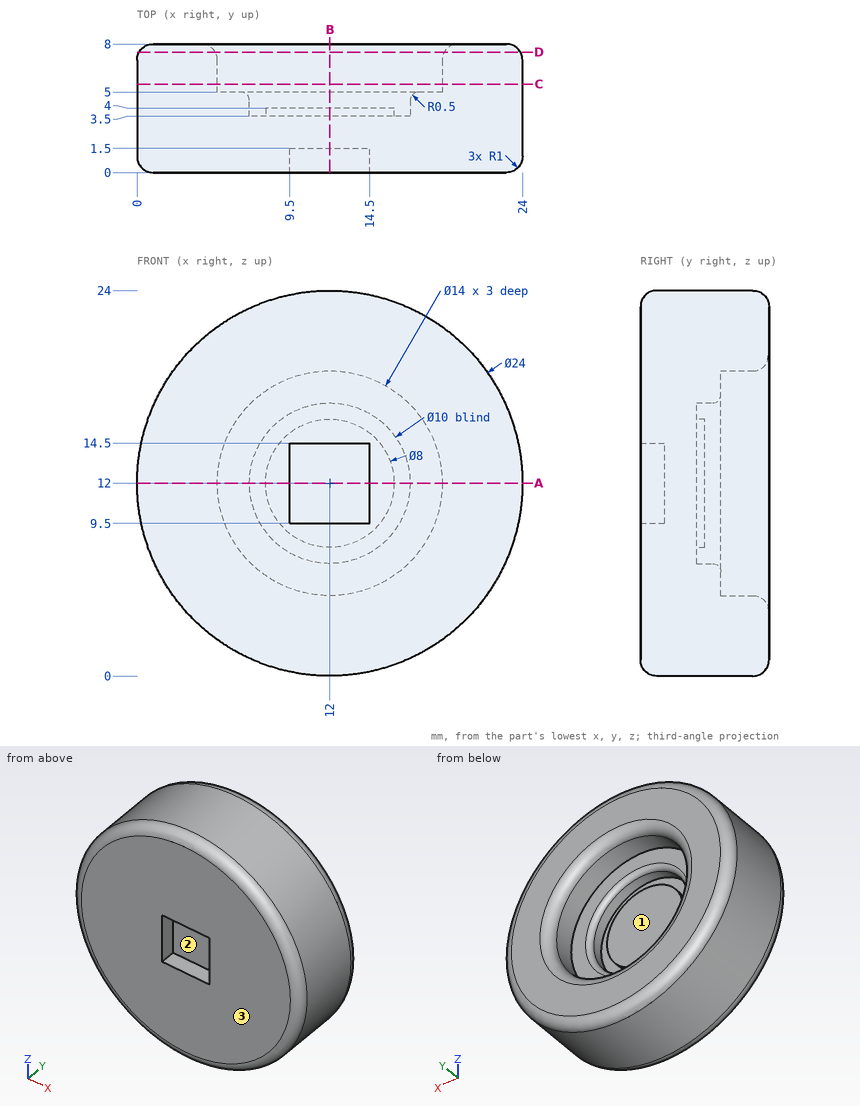
Input: dimensioned drawing with shaded views. Units: mm. Origin: part minimum x, y, z. A direction names the side the tool comes from. Coordinates: 2 decimals unless noted, no trailing zeros. Order: outer loops, then holes, each group sorted by start corner. A loop starts at its lowest first (then second) coordinate and runs counter-clockwise, first axis right, second up.
(1) Section query A-A (z = 12). Return the cut outline in (x, y), plus the area to 3 significant figures.
(2) Section query C-C (y = 5.5). Return the cut outline in (x, z), plus the area to 3 significant figures.
(3) Material intervals for probe 1 along X at (y, z) = (3.8, 12); probe 2 along Z at (x, y) = (12, 5.5), sorted ascending.
(4) Section query D-D (y = 7.5). Return the cut outline in (x, z).
(5) First-contact query: pin 1 (4 mm diameter, centred on x = 12, z = 10.5, fed in from +Y); pin 2 (2 mm diameter, centred on x = 13.5, z = 7, fed in from +Y); pin 3 (1.5 mm diameter, centred on y = 3.5, z = 17.5, fed in from +X). Flat tips, straight axial feed; report the tip coordinate or a pass-through.
(6) Access query for the marked faces 1, 2 and 3. Directions: +Z, -Z, +X, -X, +Y, -Y. A direction counts if a zero-diameter tool reaches every point of the face in a straight line with its end or side. Return the directions, or none.
(7) Section query B-B (x = 12). Return the cut outline in (y, z), plus the area to 3 significant figures.
Solution:
1. outline: (0, 1) arc R1 ccw to (1, 0) - (9.5, 0) - (9.5, 1.5) - (14.5, 1.5) - (14.5, 0) - (23, 0) arc R1 ccw to (24, 1) - (24, 7) arc R1 ccw to (23, 8) - (20, 8) arc R1 ccw to (19, 7) - (19, 5) - (17.5, 5) arc R0.5 ccw to (17, 4.5) - (17, 3.5) - (16, 3.5) - (16, 4) - (8, 4) - (8, 3.5) - (7, 3.5) - (7, 4.5) arc R0.5 ccw to (6.5, 5) - (5, 5) - (5, 7) arc R1 ccw to (4, 8) - (1, 8) arc R1 ccw to (0, 7) - close
1. area: 130 mm2
2. outline: circle Ø24 at (12, 12); hole circle Ø14 at (12, 12)
2. area: 298 mm2
3. probe 1: x = 0 to 7, 8 to 16, 17 to 24
3. probe 2: z = 0 to 5, 19 to 24
4. outline: circle Ø23.73 at (12, 12); hole circle Ø14.27 at (12, 12)
5. pin 1: stops at y = 4
5. pin 2: stops at y = 5
5. pin 3: stops at x = 23.02
6. face 1: +Y
6. face 2: -Y
6. face 3: +Z, -Z, +X, -X, -Y
7. outline: (0, 1) arc R1 ccw to (1, 0) - (7, 0) arc R1 ccw to (8, 1) - (8, 4) arc R1 ccw to (7, 5) - (5, 5) - (5, 6.5) arc R0.5 ccw to (4.5, 7) - (3.5, 7) - (3.5, 8) - (4, 8) - (4, 16) - (3.5, 16) - (3.5, 17) - (4.5, 17) arc R0.5 ccw to (5, 17.5) - (5, 19) - (7, 19) arc R1 ccw to (8, 20) - (8, 23) arc R1 ccw to (7, 24) - (1, 24) arc R1 ccw to (0, 23) - (0, 14.5) - (1.5, 14.5) - (1.5, 9.5) - (0, 9.5) - close
7. area: 130 mm2
